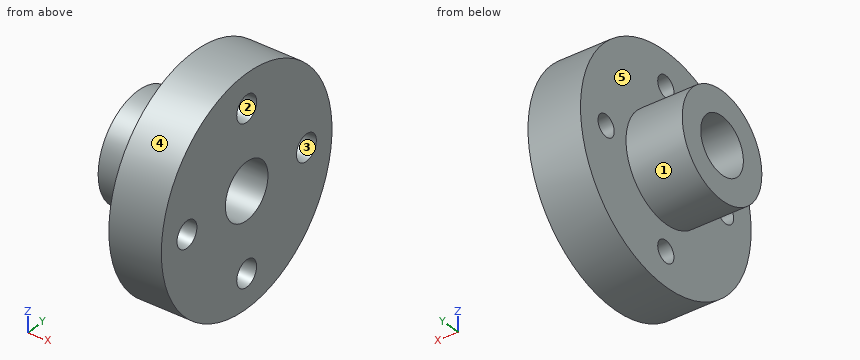
```python
from build123d import *

# Parameters (mm, degrees)
PATTERN_CIRCULAR_2_COUNT = 4


with BuildPart() as part:
    # Эскиз1 → Повернуть1 (revolve)
    with BuildSketch(Plane.XY):
        Polygon((-29, -15), (29, -15), (29, -60), (1, -60), (1, -28), (-29, -28), align=None)
    revolve(axis=Axis((-59.74315319, 0, 0), (1, 0, 0)))

    # Эскиз3 → Вырез-Повернуть1 (revolve, cut)
    with BuildSketch(Plane.XY):
        Polygon((29, 42), (1, 42), (1, 47.7), (16, 47.7), (29, 49), align=None)
    cut_revolve_1 = revolve(axis=Axis((-8.793362521, 42, 0), (1, 0, 0)), mode=Mode.SUBTRACT)

    # Круговой массив2: Вырез-Повернуть1 ×4 about axis
    pattern_circular_2_axis = Axis((0, 0, 0), (1, 0, 0))
    for i in range(1, PATTERN_CIRCULAR_2_COUNT):
        add(cut_revolve_1.rotate(pattern_circular_2_axis, i * 360 / PATTERN_CIRCULAR_2_COUNT), mode=Mode.SUBTRACT)


solid = part.part
```
Verification items for the finished model (mm, model axes). Face numbers are marked on the shaded views. A direction names the side the tool comes from. Coordinates: 2 decimals unless noted, no trailing zeros. Order: outer loops, then holes, each group sorted by start corner. A loop starts at its lowest first (then second) coordinate and runs counter-clockwise, first axis right, second up. Notation, with made-up numbers: (70, -34.5) - (77, -34.5) arc R22 cw to (77, -4.5) - close; hole circle Ø3 at (53.5, 78). An arc over 180 degrees is marked (long way). Return JSON: item names as keys, results as strings.
(1) Section check D-D, the plane x = -5. Record the cut outline in (y, z), and give its area (3 significant figures).
Filled sheet:
{"outline": "circle Ø56 at (0, 0); hole circle Ø30 at (0, 0)", "area": "1,760 mm^2"}
(2) Section check C-C, the plane z = 42. Record the cut outline in (x, y).
Filled sheet:
{"outline": "(1, -42.85) - (29, -42.85) - (29, -7) - (16, -5.7) - (1, -5.7) - close; (1, 5.7) - (16, 5.7) - (29, 7) - (29, 42.85) - (1, 42.85) - close"}
(3) Mould release check, pull along Y, two halves, no side actions. Record for the marked faces 3, 4 and 5: pulls with the +Y half, pulls with the -Y half, needs draft (parallel to the pull), parting line crosses it, or undercut.
Filled sheet:
{"face 3": "undercut", "face 4": "parting line crosses it", "face 5": "needs draft"}
(4) Go/stop test with flat-tipped pins: pin 1 (4 mm diameter, centred on x = 14, y = 30, fed in from -Z); pin 2 (7 mm diameter, centred on y = 0, z = -42, fed in from +X); pin 3 (5 mm diameter, centred on x = -19.5, z = -18, fed in from +Y); pin 4 (4 mm diameter, centred on x = 7.5, y = 28.5, fed in from -Z). Record where each tip stops, or that it passes through.
Filled sheet:
{"pin 1": "stops at z = -53.07", "pin 2": "passes through", "pin 3": "stops at y = 23.32", "pin 4": "stops at z = -53.83"}
(5) Section check A-A, the plane y = 0. Record the cut outline in (x, z).
Filled sheet:
{"outline": "(-29, -28) - (1, -28) - (1, -36.3) - (16, -36.3) - (29, -35) - (29, -15) - (-29, -15) - close; (-29, 15) - (29, 15) - (29, 35) - (16, 36.3) - (1, 36.3) - (1, 28) - (-29, 28) - close; (1, -60) - (29, -60) - (29, -49) - (16, -47.7) - (1, -47.7) - close; (1, 47.7) - (16, 47.7) - (29, 49) - (29, 60) - (1, 60) - close"}
(6) Thickness scan on line 1 along Z through (x, y) = (22, -4); line 2 along X through (y, z) = (37, 24.5); line 3 along Z through (x, y) = (12.25, 42). Record the ranges inside material, lowest first.
Filled sheet:
{"line 1": "z = -59.87 to -46.87, -37.13 to -14.46, 14.46 to 37.13, 46.87 to 59.87", "line 2": "x = 1 to 29", "line 3": "z = -42.85 to -5.7, 5.7 to 42.85"}
(7) Access from +Z, -Z, +X, -X, +Y, -Y to the whole of each face (thin tool, end or side, straight path). Record for the marked faces 1 and 2.
Filled sheet:
{"face 1": "-X", "face 2": "+X"}
